Here's how the part is built. I have some questions about the finished solid (model axes, mm). A direction names the side the tool comes from. Coordinates: 2 decimals unless noted, no trailing zeros. Order: outer loops, then holes, each group sorted by start corner. A loop starts at its lowest first (then second) coordinate and runs counter-clockwise, first axis right, second up. Notation, with made-up numbers: (84.25, 26) - (127.25, 26) arc R18 cw to (127.25, 38) - close; hole circle Ø3 at (79, -20). An arc over 180 degrees is marked (long way). Answer as CSV lines item,"result". Start each with the question number.
Item 1: Imagine slicing it at A-A on y = 17.85. List the corners of the cut face in (x, z) for me.
Item 2: I need wall thicknesses on line 1 (Y direction, x = 3.25, z = -15); line 2 (Z direction, x = 4.75, y = 24); line 3 (X direction, y = 29.7, z = -28). Which ranges of each line are inside material? Lowest first, please.
Item 3: We'd pull the mould along Z, two halves only. Please class faces 5 (the face through (2.46, 4.86, -12.9)), 6 (the face through (4, 16, -34)), 7 (the face through (0, 16, -9)), 8 (the face through (2.46, 16.82, -10.93)): pulls with the +Z half, pulls with the -Z half, needs draft (parallel to the pull), parting line crosses it, or undercut.
Item 4: On a 3-axis mill with a long thin cutter (end or side, diameter ignored), from which of +Z, -Z, +X, -X, +Y, -Y can I reach the whole of each face in a straight line? I mean faces 1 (the face through (2, 10, -12)), 2 (the face through (5.19, 30.48, -27.62)), 3 (the face through (4.27, 1.52, -29.22)), 4 (the face through (6.5, 5.9, -14.9)). Say none if no direction works.
Item 5: I'm going to push flat-ended pins straight in: pin 1 (4 mm diameter, centred on y = 20.5, z = -10, fed in from -X); pin 2 (3 mm diameter, centred on x = 4, z = -28, fed in from -Y); pin 3 (2 mm diameter, centred on x = 4, z = -6, fed in from +Y). Where does each tip first touch, or does it pass through?
Item 6: Imagine slicing it at C-C on x = 5.75. List the corners of the cut face in (y, z) for me.
Item 7: Imagine slicing it at B-B on z = -20.5. List the corners of the cut face in (x, y) for me, and give its area (3 significant figures).
from build123d import *

# Parameters (mm, degrees)
SKETCH1_W                       = 34
SKETCH1_H                       = 32
BOSS_EXTRUDE1_DEPTH             = 8
CUT_EXTRUDE1_REACH              = 49.371
SKETCH2_R                       = 6.1
SKETCH2_R_2                     = 3
SKETCH2_R_3                     = 1.5
CIRPATTERN1_OUTLINE_R           = 1.5
CIRPATTERN1_DEPTH               = 8
CUT_EXTRUDE2_DEPTH              = 5
TAP_DRILL_FOR_M3X0_5_TAP1_D     = 2.5
TAP_DRILL_FOR_M3X0_5_TAP1_DEPTH = 3
TAP_DRILL_FOR_M3X0_5_TAP1_TIP   = 0.751075774
TAP_DRILL_FOR_M3X0_5_TAP2_D     = 2.5
TAP_DRILL_FOR_M3X0_5_TAP2_DEPTH = 3
TAP_DRILL_FOR_M3X0_5_TAP2_TIP   = 0.751075774


# Read off the part's stored shape, not the designer's step: CirPattern1
with BuildPart() as part:
    # Sketch1 → Boss-Extrude1 (new body)
    with BuildSketch(Plane(origin=(0, 0, 0), x_dir=(0, 0, -1), z_dir=(1, 0, 0))):
        with Locations((17, 16)):
            Rectangle(SKETCH1_W, SKETCH1_H)
    extrude(amount=BOSS_EXTRUDE1_DEPTH)

    # Sketch2 → Cut-Extrude1 (cut, up to next)
    with BuildSketch(Plane(origin=(8, 0, 0), x_dir=(0, 0, -1), z_dir=(1, 0, 0)), mode=Mode.PRIVATE) as cut_extrude1_sk1:
        with Locations((17.681074437, 17.85)):
            Circle(SKETCH2_R)
    cut_extrude1_tool1 = extrude(cut_extrude1_sk1.sketch, amount=-CUT_EXTRUDE1_REACH, mode=Mode.PRIVATE) & part.part
    # Sketch2 → Cut-Extrude1 (cut, up to next)
    with BuildSketch(Plane(origin=(8, 0, 0), x_dir=(0, 0, -1), z_dir=(1, 0, 0)), mode=Mode.PRIVATE) as cut_extrude1_sk2:
        with Locations((6, 13.4)):
            Circle(SKETCH2_R_2)
    cut_extrude1_tool2 = extrude(cut_extrude1_sk2.sketch, amount=-CUT_EXTRUDE1_REACH, mode=Mode.PRIVATE) & part.part
    # Sketch2 → Cut-Extrude1 (cut, up to next)
    with BuildSketch(Plane(origin=(8, 0, 0), x_dir=(0, 0, -1), z_dir=(1, 0, 0)), mode=Mode.PRIVATE) as cut_extrude1_sk3:
        with Locations((27.960419941, 21.766)):
            Circle(SKETCH2_R_3)
    cut_extrude1_tool3 = extrude(cut_extrude1_sk3.sketch, amount=-CUT_EXTRUDE1_REACH, mode=Mode.PRIVATE) & part.part
    add(cut_extrude1_tool1.solids().sort_by_distance((8, 17.85, -17.681074))[0], mode=Mode.SUBTRACT)
    add(cut_extrude1_tool2.solids().sort_by_distance((8, 13.4, -6))[0], mode=Mode.SUBTRACT)
    add(cut_extrude1_tool3.solids().sort_by_distance((8, 21.766, -27.96042))[0], mode=Mode.SUBTRACT)

    # CirPattern1 outline → CirPattern1 (cut)
    with BuildSketch(Plane.YZ):
        with Locations((6.989825659, -15.932757166)):
            Circle(CIRPATTERN1_OUTLINE_R)
        with Locations((24.794174341, -9.150046203)):
            Circle(CIRPATTERN1_OUTLINE_R)
    extrude(amount=CIRPATTERN1_DEPTH, mode=Mode.SUBTRACT)

    # Sketch3 → Cut-Extrude2 (cut)
    with BuildSketch(Plane(origin=(0, 0, 0), x_dir=(0, 0, -1), z_dir=(1, 0, 0))):
        with BuildLine():
            Line((32, 25), (32, 7))
            ThreePointArc((32, 7), (31.121320344, 4.878679656), (29, 4))
            Line((29, 4), (15, 4))
            ThreePointArc((15, 4), (12.878679656, 4.878679656), (12, 7))
            Line((12, 7), (12, 13.4))
            ThreePointArc((12, 13.4), (10.898979486, 16.864101615), (8, 19.056854249))
            ThreePointArc((8, 19.056854249), (6.550510257, 20.153230567), (6, 21.885281374))
            Line((6, 21.885281374), (6, 25))
            ThreePointArc((6, 25), (6.878679656, 27.121320344), (9, 28))
            Line((9, 28), (29, 28))
            ThreePointArc((29, 28), (31.121320344, 27.121320344), (32, 25))
        make_face()
    extrude(amount=CUT_EXTRUDE2_DEPTH, mode=Mode.SUBTRACT)

    # Tap Drill for M3x0.5 Tap1
    with Locations(Plane(origin=(0, 32, 0), x_dir=(-1, 0, 0), z_dir=(0, 1, 0))):
        with Locations((-4, -6), (-4, -28)):
            Hole(TAP_DRILL_FOR_M3X0_5_TAP1_D / 2, depth=TAP_DRILL_FOR_M3X0_5_TAP1_DEPTH)
            with Locations((0, 0, -(TAP_DRILL_FOR_M3X0_5_TAP1_DEPTH + TAP_DRILL_FOR_M3X0_5_TAP1_TIP / 2))):  # 118° drill point
                Cone(0, TAP_DRILL_FOR_M3X0_5_TAP1_D / 2, TAP_DRILL_FOR_M3X0_5_TAP1_TIP, mode=Mode.SUBTRACT)

    # Tap Drill for M3x0.5 Tap2
    with Locations(Plane.XZ):
        with Locations((4, -6), (4, -28)):
            Hole(TAP_DRILL_FOR_M3X0_5_TAP2_D / 2, depth=TAP_DRILL_FOR_M3X0_5_TAP2_DEPTH)
            with Locations((0, 0, -(TAP_DRILL_FOR_M3X0_5_TAP2_DEPTH + TAP_DRILL_FOR_M3X0_5_TAP2_TIP / 2))):  # 118° drill point
                Cone(0, TAP_DRILL_FOR_M3X0_5_TAP2_D / 2, TAP_DRILL_FOR_M3X0_5_TAP2_TIP, mode=Mode.SUBTRACT)


solid = part.part
Responses:
1,outline,"(0, -34) - (8, -34) - (8, -23.78) - (5, -23.78) - (5, -32) - (0, -32) - close; (0, -10.02) - (5, -10.02) - (5, -11.58) - (8, -11.58) - (8, 0) - (0, 0) - close"
2,line 1,"y = 0 to 4, 28 to 32"
2,line 2,"z = -34 to -32, -6 to 0"
2,line 3,"x = 0 to 2.75, 5.25 to 8"
3,face 5,"undercut"
3,face 6,"pulls with the -Z half"
3,face 7,"needs draft"
3,face 8,"undercut"
4,face 1,"-X"
4,face 2,"+Y"
4,face 3,"-Y"
4,face 4,"+X, -X"
5,pin 1,"stops at x = 5"
5,pin 2,"stops at y = 0"
5,pin 3,"stops at y = 28.85"
6,outline,"(0, -34) - (32, -34) - (32, 0) - (0, 0) - close; hole circle Ø3 at (6.99, -15.93); hole circle Ø6 at (13.4, -6); hole circle Ø12.2 at (17.85, -17.68); hole circle Ø3 at (21.77, -27.96); hole circle Ø3 at (24.79, -9.15)"
7,outline,"(0, 0) - (8, 0) - (8, 12.44) - (5, 12.44) - (5, 4) - (0, 4) - close; (0, 28) - (5, 28) - (5, 23.26) - (8, 23.26) - (8, 32) - (0, 32) - close"
7,area,"104 mm^2"
